Read the model definition and answer for the solid it produces. Units are mm, in the model's axes. Give positions to 0.01 mm unless a question says otherwise; leave off trailing zeros. Loops run counter-clockwise (first coordinate to the right, second up) from the corner with the lowest first, then second, coordinate; pieces in that order, holes last. Notation, with made-up numbers: (79, -33.5) - (124, -33.5) arc R11 cw to (124, -24.5) - close; hole circle Ø5 at (-0.75, -12.5). An arc over 180 degrees is marked (long way). Put each result on its own line as item: value. Start each with the question number.
1. A cutting plane is placed at B-B, the plane z = 0. Determine the outline of the cut face in (x, y).
2. Given pin 1 Ø10 at (x, z) = (23.5, 29) entering from +Y, flat-ended and moving along its own axis, determine where the tip first touches the part or whether it passes through.
3. A cutting plane is placed at A-A, the plane x = 0. Determine the outline of the cut face in (y, z), plus the area to 3 significant figures.
4. Consider L1, parallel to Z at x = 0, y = -26; L2, parallel to X at y = -13, z = 0.5; L3, parallel to X at y = -21, z = 10. Determine where each line is inside the solid, lowest interval first. Write a range as from..to.
5. For a pull along Z with two mould halves and no side action, classify faces 1 (the cylindrical face through (-0.587, -1.449, -36.492)), 2 (the cylindrical face through (45.485, -38.562, 36.571)), 3 (the cylindrical face through (-45.485, -1.449, -0.461)), 4 (the cylindrical face through (5.868, -37.567, -26.424)) as released by +Z, released by -Z, zero draft, split by the parting line, or undercut.
6. A cutting plane is placed at C-C, the plane y = -10.5. Determine the outline of the cut face in (x, z).
```python
from build123d import *

# Parameters (mm, degrees)
F0_W         = 94.0244570374
F0_H         = 76.03880018
F1_DEPTH     = 76.2
F2_R         = 27.0679011962
F3_DEPTH     = 101.6
F4_R         = 5.08
F5_T1_DEPTH  = 83.8644570374
F5_T3_DEPTH  = 65.87880018
F5_T5_DEPTH  = 66.04
F5_S9_W      = 5.08
F5_S9_H      = 5.08
F5_T10_DEPTH = 5.08
F5_S15_W     = 5.08
F5_S15_H     = 5.08
F5_T16_DEPTH = 5.08
F5_S21_W     = 5.08
F5_S21_H     = 5.08
F5_T22_DEPTH = 5.08
F5_S27_W     = 5.08
F5_S27_H     = 5.08
F5_T28_DEPTH = 5.08


# Not quite as in the source:
# - a fillet or chamfer that OpenCascade refuses, or shapes differently, is made with other operations: its cross-section is extruded or revolved along the edge and cut away or added


with BuildPart() as f1:
    # F0 (on Front) → F1 (new body)
    with BuildSketch(Plane.XZ):
        Rectangle(F0_W, F0_H)
    extrude(amount=F1_DEPTH)

    # F2 (on face) → F3 (cut)
    with BuildSketch(Plane(origin=(0, 0, 0), x_dir=(-1, 0, 0), z_dir=(0, 1, 0))):
        Circle(F2_R)
    extrude(amount=-F3_DEPTH, mode=Mode.SUBTRACT)

    # F4
    f4_edges = [f1.edges().sort_by_distance(p)[0] for p in [
        (0, -76.2, 38.0194),
        (47.012229, -38.1, 38.0194),
        (0, 0, 38.0194),
        (-47.012229, -38.1, 38.0194),
        (47.012229, -76.2, 0),
        (47.012229, 0, 0),
        (47.012229, -38.1, -38.0194),
        (0, -76.2, -38.0194),
        (-47.012229, -76.2, 0),
    ]]
    fillet(f4_edges, radius=F4_R)

    # F5: fillet of radius 5.08 on 3 edges, made by hand

    # F5_s2 → F5_t1 (cut)
    with BuildSketch(Plane.YZ.offset(-41.9322285187)):
        with BuildLine():
            ThreePointArc((0, -32.93940009), (-1.4878975516, -36.5315025384), (-5.08, -38.01940009))
            Line((-5.08, -38.01940009), (0, -38.01940009))
            Line((0, -38.01940009), (0, -32.93940009))
        make_face()
    extrude(amount=F5_T1_DEPTH, mode=Mode.SUBTRACT)

    # F5_s4 → F5_t3 (cut)
    with BuildSketch(Plane.XY.offset(-32.93940009)):
        with BuildLine():
            ThreePointArc((-41.9322285187, 0), (-45.5243309672, -1.4878975516), (-47.0122285187, -5.08))
            Line((-47.0122285187, -5.08), (-47.0122285187, 0))
            Line((-47.0122285187, 0), (-41.9322285187, 0))
        make_face()
    extrude(amount=F5_T3_DEPTH, mode=Mode.SUBTRACT)

    # F5_s6 → F5_t5 (cut)
    with BuildSketch(Plane.XZ.offset(5.08)):
        with BuildLine():
            ThreePointArc((-41.9322285187, -38.01940009), (-45.5243309672, -36.5315025384), (-47.0122285187, -32.93940009))
            Line((-47.0122285187, -32.93940009), (-47.0122285187, -38.01940009))
            Line((-47.0122285187, -38.01940009), (-41.9322285187, -38.01940009))
        make_face()
    extrude(amount=F5_T5_DEPTH, mode=Mode.SUBTRACT)


with BuildPart() as f5_tool8:
    # F5_s9 → F5_t10 (new body)
    with BuildSketch(Plane.XY.offset(-32.93940009)):
        with Locations((-44.4722285187, -73.66)):
            Rectangle(F5_S9_W, F5_S9_H)
    extrude(amount=-F5_T10_DEPTH)

    # F5_s11 → F5_t12 (revolve, cut)
    with BuildSketch(Plane(origin=(-41.9322285187, -71.12, -32.93940009), x_dir=(0.7071067812, 0.7071067812, 0), z_dir=(-0.7071067812, 0.7071067812, 0))):
        with BuildLine():
            ThreePointArc((0, -5.08), (5.08, 0), (0, 5.08))
            Line((0, 5.08), (0, -5.08))
        make_face()
    revolve(axis=Axis((-41.9322285187, -71.12, -32.93940009), (0, 0, -1)), mode=Mode.SUBTRACT)


with BuildPart() as f1_1:
    add(f1.part)

    # F5_t7: cut F5_tool8
    add(f5_tool8.part, mode=Mode.SUBTRACT)


with BuildPart() as f5_tool14:
    # F5_s15 → F5_t16 (new body)
    with BuildSketch(Plane.XZ.offset(5.08)):
        with Locations((-44.4722285187, 35.47940009)):
            Rectangle(F5_S15_W, F5_S15_H)
    extrude(amount=-F5_T16_DEPTH)

    # F5_s17 → F5_t18 (revolve, cut)
    with BuildSketch(Plane(origin=(-41.9322285187, -5.08, 32.93940009), x_dir=(0.7071067812, 0, -0.7071067812), z_dir=(0.7071067812, 0, 0.7071067812))):
        with BuildLine():
            ThreePointArc((0, -5.08), (5.08, 0), (0, 5.08))
            Line((0, 5.08), (0, -5.08))
        make_face()
    revolve(axis=Axis((-41.9322285187, -5.08, 32.93940009), (0, 1, 0)), mode=Mode.SUBTRACT)


with BuildPart() as f1_2:
    add(f1_1.part)

    # F5_t13: cut F5_tool14
    add(f5_tool14.part, mode=Mode.SUBTRACT)


with BuildPart() as f5_tool20:
    # F5_s21 → F5_t22 (new body)
    with BuildSketch(Plane.XZ.offset(5.08)):
        with Locations((44.4722285187, -35.47940009)):
            Rectangle(F5_S21_W, F5_S21_H)
    extrude(amount=-F5_T22_DEPTH)

    # F5_s23 → F5_t24 (revolve, cut)
    with BuildSketch(Plane(origin=(41.9322285187, -5.08, -32.93940009), x_dir=(-0.7071067812, 0, 0.7071067812), z_dir=(-0.7071067812, 0, -0.7071067812))):
        with BuildLine():
            ThreePointArc((0, -5.08), (5.08, 0), (0, 5.08))
            Line((0, 5.08), (0, -5.08))
        make_face()
    revolve(axis=Axis((41.9322285187, -5.08, -32.93940009), (0, 1, 0)), mode=Mode.SUBTRACT)


with BuildPart() as f1_3:
    add(f1_2.part)

    # F5_t19: cut F5_tool20
    add(f5_tool20.part, mode=Mode.SUBTRACT)


with BuildPart() as f5_tool26:
    # F5_s27 → F5_t28 (new body)
    with BuildSketch(Plane.XZ.offset(5.08)):
        with Locations((-44.4722285187, -35.47940009)):
            Rectangle(F5_S27_W, F5_S27_H)
    extrude(amount=-F5_T28_DEPTH)

    # F5_s29 → F5_t30 (revolve, cut)
    with BuildSketch(Plane(origin=(-41.9322285187, -5.08, -32.93940009), x_dir=(0.7071067812, 0, 0.7071067812), z_dir=(-0.7071067812, 0, 0.7071067812))):
        with BuildLine():
            ThreePointArc((0, -5.08), (5.08, 0), (0, 5.08))
            Line((0, 5.08), (0, -5.08))
        make_face()
    revolve(axis=Axis((-41.9322285187, -5.08, -32.93940009), (0, 1, 0)), mode=Mode.SUBTRACT)


with BuildPart() as f1_4:
    add(f1_3.part)

    # F5_t25: cut F5_tool26
    add(f5_tool26.part, mode=Mode.SUBTRACT)


solid = f1_4.part
```
Return value:
1. outline: (-47.01, -71.12) arc R5.08 ccw to (-41.93, -76.2) - (-27.07, -76.2) - (-27.07, 0) - (-41.93, 0) arc R5.08 ccw to (-47.01, -5.08) - close; (27.07, -76.2) - (41.93, -76.2) arc R5.08 ccw to (47.01, -71.12) - (47.01, -5.08) arc R5.08 ccw to (41.93, 0) - (27.07, 0) - close
2. pin 1: stops at y = 0
3. outline: (-76.2, -32.94) arc R5.08 ccw to (-71.12, -38.02) - (-5.08, -38.02) arc R5.08 ccw to (0, -32.94) - (0, -27.07) - (-76.2, -27.07) - close; (-76.2, 27.07) - (0, 27.07) - (0, 32.94) arc R5.08 ccw to (-5.08, 38.02) - (-71.12, 38.02) arc R5.08 ccw to (-76.2, 32.94) - close
3. area: 1,650 mm2
4. L1: z = -38.02..-27.07, 27.07..38.02
4. L2: x = -47.01..-27.06, 27.06..47.01
4. L3: x = -47.01..-25.15, 25.15..47.01
5. face 1: released by -Z
5. face 2: released by +Z
5. face 3: zero draft
5. face 4: undercut
6. outline: (-47.01, -32.94) arc R5.08 ccw to (-41.93, -38.02) - (41.93, -38.02) arc R5.08 ccw to (47.01, -32.94) - (47.01, 32.94) arc R5.08 ccw to (41.93, 38.02) - (-41.93, 38.02) arc R5.08 ccw to (-47.01, 32.94) - close; hole circle Ø54.14 at (0, 0)
